from build123d import *

# Parameters (mm, degrees)
SKETCH1_W           = 19
SKETCH1_H           = 9
BOSS_EXTRUDE1_DEPTH = 4
CUT_EXTRUDE1_REACH  = 10
SKETCH2_W           = 15
SKETCH2_H           = 7
CUT_EXTRUDE3_REACH  = 10
SKETCH5_W           = 2
SKETCH5_H           = 9
BOSS_EXTRUDE2_DEPTH = 5
CUT_EXTRUDE4_REACH  = 19
SKETCH7_W           = 8
SKETCH7_H           = 2
SKETCH8_R           = 0.375
CUT_EXTRUDE6_DEPTH  = 8
SKETCH9_W           = 2
SKETCH9_H           = 7.24
BOSS_EXTRUDE3_DEPTH = 8
CUT_EXTRUDE7_REACH  = 4


with BuildPart() as part:
    # Sketch1 → Boss-Extrude1 (new body, symmetric)
    with BuildSketch(Plane.XY):
        Rectangle(SKETCH1_W, SKETCH1_H)
    extrude(amount=BOSS_EXTRUDE1_DEPTH, both=True)

    # Sketch2 → Cut-Extrude1 (cut, up to next)
    with BuildSketch(Plane.XY.offset(4), mode=Mode.PRIVATE) as cut_extrude1_sk1:
        with Locations((0, -1)):
            Rectangle(SKETCH2_W, SKETCH2_H)
    cut_extrude1_tool1 = extrude(cut_extrude1_sk1.sketch, amount=-CUT_EXTRUDE1_REACH, mode=Mode.PRIVATE) & part.part
    add(cut_extrude1_tool1.solids().sort_by_distance((0, -1, 4))[0], mode=Mode.SUBTRACT)

    # Sketch5 → Cut-Extrude3 (cut, up to next)
    with BuildSketch(Plane.XY.offset(4), mode=Mode.PRIVATE) as cut_extrude3_sk1:
        with Locations((8.5, 0)):
            Rectangle(SKETCH5_W, SKETCH5_H)
    cut_extrude3_tool1 = extrude(cut_extrude3_sk1.sketch, amount=-CUT_EXTRUDE3_REACH, mode=Mode.PRIVATE) & part.part
    add(cut_extrude3_tool1.solids().sort_by_distance((8.5, 0, 4))[0], mode=Mode.SUBTRACT)

    # Sketch6 → Boss-Extrude2 (add)
    with BuildSketch(Plane(origin=(-7.5, 0, 0), x_dir=(0, 0, -1), z_dir=(1, 0, 0))):
        Polygon((4, 2.5), (1.25, 2.5), (2, 0.999999988), (2.249999998, 0.499999988), (-2.249999998, 0.499999988), (-2, 0.999999988), (-1.25, 2.5), (-4, 2.5), (-4, -0.260952874), (4, -0.260952874), align=None)
    extrude(amount=BOSS_EXTRUDE2_DEPTH)

    # Sketch7 → Cut-Extrude4 (cut, up to next)
    with BuildSketch(Plane(origin=(7.5, 0, 0), x_dir=(0, 0, -1), z_dir=(1, 0, 0)), mode=Mode.PRIVATE) as cut_extrude4_sk1:
        with Locations((0, 3.5)):
            Rectangle(SKETCH7_W, SKETCH7_H)
    cut_extrude4_tool1 = extrude(cut_extrude4_sk1.sketch, amount=-CUT_EXTRUDE4_REACH, mode=Mode.PRIVATE) & part.part
    add(cut_extrude4_tool1.solids().sort_by_distance((7.5, 3.5, 0))[0], mode=Mode.SUBTRACT)

    # Sketch8 → Cut-Extrude6 (cut)
    with BuildSketch(Plane(origin=(0, 0, -4), x_dir=(-1, 0, 0), z_dir=(0, 0, -1))):
        with Locations((5.019927309, 1.462821702)):
            Circle(SKETCH8_R)
    extrude(amount=-CUT_EXTRUDE6_DEPTH, mode=Mode.SUBTRACT)

    # Sketch9 → Boss-Extrude3 (add)
    with BuildSketch(Plane(origin=(0, 0, -4), x_dir=(-1, 0, 0), z_dir=(0, 0, -1))):
        with Locations((8.5, -3.880952874)):
            Rectangle(SKETCH9_W, SKETCH9_H)
    extrude(amount=-BOSS_EXTRUDE3_DEPTH)

    # Sketch10 → Cut-Extrude7 (cut, up to next)
    with BuildSketch(Plane(origin=(-7.5, 0, 0), x_dir=(0, 0, -1), z_dir=(1, 0, 0)), mode=Mode.PRIVATE) as cut_extrude7_sk1:
        Polygon((-2.249999998, 0.499999988), (-1.25, 2.5), (1.25, 2.5), (2.249999998, 0.499999988), align=None)
    cut_extrude7_tool1 = extrude(cut_extrude7_sk1.sketch, amount=-CUT_EXTRUDE7_REACH, mode=Mode.PRIVATE) & part.part
    add(cut_extrude7_tool1.solids().sort_by_distance((-7.5, 1.404762, 0))[0], mode=Mode.SUBTRACT)


solid = part.part
The listing builds one solid part. Answer for the finished solid, in the listing's coordinates (mm). A direction names the side the tool comes from. Round coordinates to 2 decimals unless told otherwise and drop trailing zeros. Order: outer loops, then holes, each group sorted by start corner. A loop starts at its lowest first (then second) coordinate and runs counter-clockwise, first axis right, second up. Notation, with made-up numbers: (65, 59) - (113, 59) arc R19 ccw to (113, 78) - close; hole circle Ø6 at (29.5, -21.75). An arc over 180 degrees is marked (long way). Write item = value, one per line. Start each with the question number.
1) For a pull along Z with two mould halves and no side action, classify faces 4 (the flat face through (-8, -1, -4)), 5 (the flat face through (-6, 0.5, 0)), 6 (the flat face through (-7.5, -4, 0)) as released by +Z, released by -Z, zero draft, split by the parting line, or undercut.
2) Section B-B, the plane x = -5.25 is taken. Write down the section's boundary in (y, z), plus the area to 3 significant figures.
3) Section A-A, the plane z = -2 is taken. Write down the section's boundary in (x, y) (3 decimals).
4) For faces 1 (the flat face through (-8, -7.501, 0)), 2 (the flat face through (-5.951, 1.514, -1.743)), 3 (the flat face through (-5, -0.261, 0)), determine the directions among +Z, -Z, +X, -X, +Y, -Y from which every point of the face is accessible in a straight line to the end or side of a thin tool.
5) Straight lines are drawn through the part: L1, parallel to Y at x = -4, z = -0.5; L2, parallel to X at y = -1.25, z = 3; L3, parallel to Y at x = -3.5, z = 2. For each, find the intervals that lie inside material, in ascending order.
6) Section D-D, the plane z = 1 is taken. Write down the section's boundary in (x, y), plus the area to 3 significant figures.
7) Section C-C, the plane x = -4 is taken. Write down the section's boundary in (y, z).
8) Given pin 1 (2.5 mm diameter, centred on x = -4, z = -0.5, fed in from -Y); pin 2 (3.5 mm diameter, centred on x = -6, z = 0, fed in from +Y); pin 3 (3 mm diameter, centred on y = -2.5, z = -2.5, fed in from +X), each flat-ended and moving along its own axis, determine where each tip first touches the part or whether it passes through.
Results list:
q1.face_4 = released by -Z
q1.face_5 = undercut
q1.face_6 = zero draft
q2.outline = (-0.26, -4) - (1.17, -4) - (1.17, -1.92) - (0.5, -2.25) - (0.5, 2.25) - (1.17, 1.92) - (1.17, 4) - (-0.26, 4) - close; (1.76, -4) - (2.5, -4) - (2.5, -1.25) - (1.76, -1.62) - close; (1.76, 1.62) - (2.5, 1.25) - (2.5, 4) - (1.76, 4) - close
q2.area = 12.4 mm^2
q3.outline = (-9.5, -7.501) - (-7.5, -7.501) - (-7.5, -0.261) - (-2.5, -0.261) - (-2.5, 0.5) - (-9.5, 0.5) - close; (-9.5, 1) - (-2.5, 1) - (-2.5, 2.5) - (-9.5, 2.5) - close; hole circle Ø0.75 at (-5.02, 1.463)
q4.face_1 = +Z, -Z, +X, -X, -Y
q4.face_2 = +X, -X
q4.face_3 = +Z, -Z, +X, -Y
q5.L1 = -0.26 to 0.5
q5.L2 = -9.5 to -7.5
q5.L3 = -0.26 to 0.5, 1 to 2.5
q6.outline = (-9.5, -7.5) - (-7.5, -7.5) - (-7.5, -0.26) - (-2.5, -0.26) - (-2.5, 0.5) - (-9.5, 0.5) - close
q6.area = 19.8 mm^2
q7.outline = (-0.26, -4) - (2.5, -4) - (2.5, -1.25) - (0.5, -2.25) - (0.5, 2.25) - (2.5, 1.25) - (2.5, 4) - (-0.26, 4) - close
q8.pin_1 = -0.26
q8.pin_2 = 2.5
q8.pin_3 = -7.5
